```python
from build123d import *

# Parameters (mm, degrees)
SKETCH1_R               = 10
BOSS_EXTRUDE1_DEPTH     = 10
SKETCH2_W               = 25
SKETCH2_H               = 50
BOSS_EXTRUDE2_DEPTH     = 5
SKETCH3_W               = 25
SKETCH3_H               = 50
BOSS_EXTRUDE3_DEPTH     = 5
SKETCH4_W               = 5
SKETCH4_H               = 40
BOSS_EXTRUDE4_DEPTH     = 40
SKETCH5_R               = 5
CUT_EXTRUDE1_DEPTH      = 1
CUT_EXTRUDE1_DEPTH_BACK = 41
FILLET1_R               = 10


with BuildPart() as part:
    # Sketch1 → Boss-Extrude1 (new body)
    with BuildSketch(Plane(origin=(0, 0, 0), x_dir=(1, 0, 0), z_dir=(0, 1, 0))):
        with BuildLine():
            Line((-22.5, 15), (2.5, 15))
            Line((2.5, 15), (2.5, -15))
            Line((2.5, -15), (-22.5, -15))
            Line((-22.5, -15), (-22.5, -20))
            Line((-22.5, -20), (22.5, -20))
            ThreePointArc((22.5, -20), (42.5, 0), (22.5, 20))
            Line((22.5, 20), (-22.5, 20))
            Line((-22.5, 20), (-22.5, 15))
        make_face()
        with Locations((22.5, 0)):
            Circle(SKETCH1_R, mode=Mode.SUBTRACT)
    extrude(amount=BOSS_EXTRUDE1_DEPTH)

    # Sketch2 → Boss-Extrude2 (add)
    with BuildSketch(Plane(origin=(0, 0, -20), x_dir=(-1, 0, 0), z_dir=(0, 0, -1))):
        with Locations((10, 25)):
            Rectangle(SKETCH2_W, SKETCH2_H)
    extrude(amount=-BOSS_EXTRUDE2_DEPTH)

    # Sketch3 → Boss-Extrude3 (add)
    with BuildSketch(Plane.XY.offset(20)):
        with Locations((-10, 25)):
            Rectangle(SKETCH3_W, SKETCH3_H)
    extrude(amount=-BOSS_EXTRUDE3_DEPTH)

    # Sketch4 → Boss-Extrude4 (add)
    with BuildSketch(Plane.XY.offset(20)):
        with Locations((5, 30)):
            Rectangle(SKETCH4_W, SKETCH4_H)
    extrude(amount=-BOSS_EXTRUDE4_DEPTH)

    # Sketch5 → Cut-Extrude1 (cut, two sides)
    with BuildSketch(Plane.XY.offset(20)) as cut_extrude1_sk:
        with Locations((-12.5, 40)):
            Circle(SKETCH5_R)
        with Locations((-12.5, 10)):
            Circle(SKETCH5_R)
    extrude(amount=CUT_EXTRUDE1_DEPTH, mode=Mode.SUBTRACT)
    extrude(cut_extrude1_sk.sketch, amount=-CUT_EXTRUDE1_DEPTH_BACK, mode=Mode.SUBTRACT)

    # Fillet1
    fillet1_edges = [part.edges().sort_by_distance(p)[0] for p in [
        (-22.5, 0, -17.5),
        (-22.5, 50, -17.5),
        (-22.5, 50, 17.5),
        (-22.5, 0, 17.5),
    ]]
    fillet(fillet1_edges, radius=FILLET1_R)


solid = part.part
```
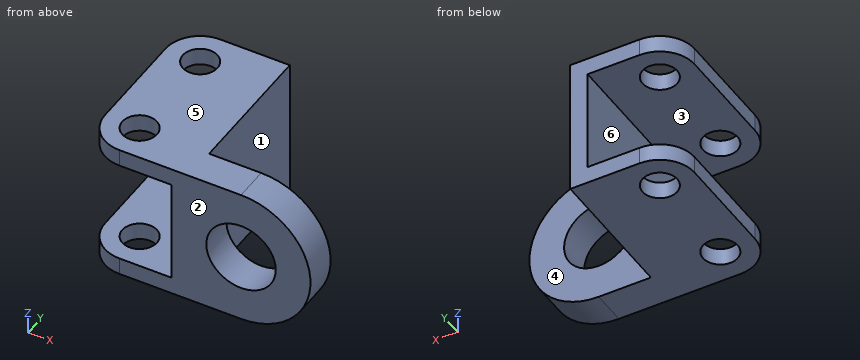
Geometry check sheet. Reference: the model listing, model coordinates, mm. Face numbers are marked on the shaded views. A direction names the side the tool comes from. Round coordinates to 2 decimals unless told otherwise and drop trailing zeros. Loops run counter-clockwise (first coordinate to the right, second up) from the corner with the lowest first, then second, coordinate; pieces in that order, holes last. Notation, with made-up numbers: M 29,-21 L 43,-21 A5 cw 43,-14 Z; hole C 68,-16.5 d9. An arc over 180 degrees is marked long. Return JSON: item names as keys, results as strings. Group by question number.
(1) Mould release check, pull along Z, two halves, no side actions. Record for the marked faces 4, 5 and 6: pulls with the +Z half, pulls with the -Z half, needs draft (parallel to the pull), parting line crosses it, or undercut.
(2) Scan lines: line 1 along Y through (x, z) = (-12.5, 17.9); line 2 along Z through (x, y) = (-0.5, 35); line 3 along Y through (x, z) = (24, -14.5). Record each from-to range of solid material in increasing order. Write a range as [from, to].
(3) Go/stop test with flat-tipped pins: pin 1 (3 mm diameter, centred on y = 38.5, z = -2.5, fed in from +X); pin 2 (6 mm diameter, centred on x = 30, y = 10, fed in from -Z); pin 3 (6 mm diameter, centred on x = -12.5, y = 40, fed in from +Z); pin 4 (1.5 mm diameter, centred on y = 10, z = -9, fed in from -X). Record where each tip stops, or that it passes through.
(4) Section check A-A, the plane y = 41. Enter the section's corners in (x, z).
(5) Section check C-C, the plane z = -3. Enter the section's corners in (x, y).
(6) Set-up check for the marked faces 1, 2 and 3: record each of +Z, -Z, +X, -X, +Y, -Y from which the full face is reachable in a straight line by a thin tool's end or side.
(7) Section check D-D, the plane y = 33. Enter the section's corners in (x, z).
(8) Section check B-B, the plane x = -2. Enter the section's corners in (y, z), and give its area (3 significant figures).
Data:
{
 "1": {"face 4": "needs draft", "face 5": "pulls with the +Z half", "face 6": "undercut"},
 "2": {"line 1": "[0, 5], [15, 35], [45, 50]", "line 2": "[-20, -15], [15, 20]", "line 3": "[0, 10]"},
 "3": {"pin 1": "x = 7.5", "pin 2": "z = -19.49", "pin 3": "through", "pin 4": "x = 2.5"},
 "4": {"outline": "M -22.45,-20 L -17.4,-20 L -17.4,-15 L -22.45,-15 Z; M -22.45,15 L -17.4,15 L -17.4,20 L -22.45,20 Z; M -7.6,-20 L 7.5,-20 L 7.5,20 L -7.6,20 L -7.6,15 L 2.5,15 L 2.5,-15 L -7.6,-15 Z"},
 "5": {"outline": "M 2.5,0 L 12.96,0 L 12.96,10 L 7.5,10 L 7.5,50 L 2.5,50 Z; M 32.04,0 L 42.27,0 L 42.27,10 L 32.04,10 Z"},
 "6": {"face 1": "+Z, -Z, +X, +Y", "face 2": "+Z, -Z, +X, -X, -Y", "face 3": "-X, +Y, -Y"},
 "7": {"outline": "M -22.5,-20 L 7.5,-20 L 7.5,20 L -22.5,20 L -22.5,15 L 2.5,15 L 2.5,-15 L -22.5,-15 Z"},
 "8": {"outline": "M 0,-20 L 50,-20 L 50,-15 L 0,-15 Z; M 0,15 L 50,15 L 50,20 L 0,20 Z", "area": "500 mm²"}
}
